Design review of the part built by this model. Coordinates are the model's own, in mm. Coordinates: 2 decimals unless noted, no trailing zeros. Order: outer loops, then holes, each group sorted by start corner. A loop starts at its lowest first (then second) coordinate and runs counter-clockwise, first axis right, second up. Notation, with made-up numbers: M -15.75,77 L 9.25,77 A20 ccw 9.25,99 Z; hole C 12.5,-29.75 d6. An arc over 180 degrees is marked long. Answer in a Markdown table with one row per item.
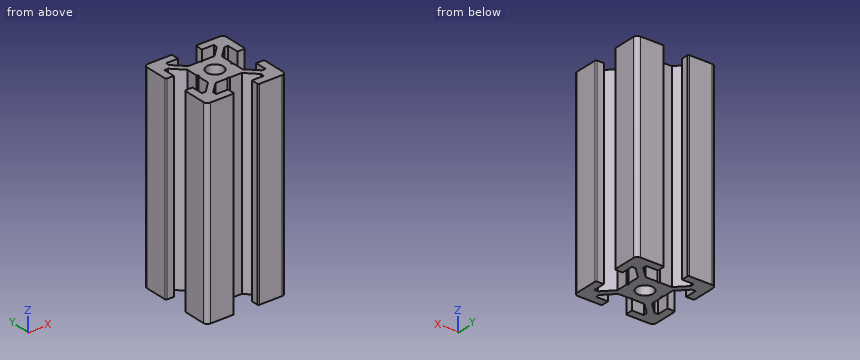
from build123d import *

# Parameters (mm, degrees)
SKETCH1_R           = 2.1
BOSS_EXTRUDE1_DEPTH = 50


with BuildPart() as part:
    # Sketch1 → Boss-Extrude1 (new body)
    with BuildSketch(Plane.XY):
        with BuildLine():
            Line((3.3, 4.360660172), (6.000039828, 7.0607))
            Line((6.000039828, 7.0607), (6.000039828, 8))
            Line((6.000039828, 8), (3.000039828, 8))
            Line((3.000039828, 8), (3.000039828, 9.7))
            ThreePointArc((3.000039828, 9.7), (3.087907794, 9.912132034), (3.300039828, 10))
            Line((3.300039828, 10), (9, 10))
            ThreePointArc((9, 10), (9.707106781, 9.707106781), (10, 9))
            Line((10, 9), (10, 3.300039828))
            ThreePointArc((10, 3.300039828), (9.912132034, 3.087907794), (9.7, 3.000039828))
            Line((9.7, 3.000039828), (8, 3.000039828))
            Line((8, 3.000039828), (8, 6.000039828))
            Line((8, 6.000039828), (7.0607, 6.000039828))
            Line((7.0607, 6.000039828), (4.360660172, 3.3))
            Line((4.360660172, 3.3), (4.360660172, 0.3))
            Line((4.360660172, 0.3), (4.060660172, 0))
            Line((4.060660172, 0), (4.360660172, -0.3))
            Line((4.360660172, -0.3), (4.360660172, -3.3))
            Line((4.360660172, -3.3), (7.0607, -6.000039828))
            Line((7.0607, -6.000039828), (8, -6.000039828))
            Line((8, -6.000039828), (8, -3.000039828))
            Line((8, -3.000039828), (9.7, -3.000039828))
            ThreePointArc((9.7, -3.000039828), (9.912132034, -3.087907794), (10, -3.300039828))
            Line((10, -3.300039828), (10, -9))
            ThreePointArc((10, -9), (9.707106781, -9.707106781), (9, -10))
            Line((9, -10), (3.300039828, -10))
            ThreePointArc((3.300039828, -10), (3.087907794, -9.912132034), (3.000039828, -9.7))
            Line((3.000039828, -9.7), (3.000039828, -8))
            Line((3.000039828, -8), (6.000039828, -8))
            Line((6.000039828, -8), (6.000039828, -7.0607))
            Line((6.000039828, -7.0607), (3.3, -4.360660172))
            Line((3.3, -4.360660172), (0.3, -4.360660172))
            Line((0.3, -4.360660172), (0, -4.060660172))
            Line((0, -4.060660172), (-0.3, -4.360660172))
            Line((-0.3, -4.360660172), (-3.3, -4.360660172))
            Line((-3.3, -4.360660172), (-6.000039828, -7.0607))
            Line((-6.000039828, -7.0607), (-6.000039828, -8))
            Line((-6.000039828, -8), (-3.000039828, -8))
            Line((-3.000039828, -8), (-3.000039828, -9.7))
            ThreePointArc((-3.000039828, -9.7), (-3.087907794, -9.912132034), (-3.300039828, -10))
            Line((-3.300039828, -10), (-9, -10))
            ThreePointArc((-9, -10), (-9.707106781, -9.707106781), (-10, -9))
            Line((-10, -9), (-10, -3.300039828))
            ThreePointArc((-10, -3.300039828), (-9.912132034, -3.087907794), (-9.7, -3.000039828))
            Line((-9.7, -3.000039828), (-8, -3.000039828))
            Line((-8, -3.000039828), (-8, -6.000039828))
            Line((-8, -6.000039828), (-7.0607, -6.000039828))
            Line((-7.0607, -6.000039828), (-4.360660172, -3.3))
            Line((-4.360660172, -3.3), (-4.360660172, -0.3))
            Line((-4.360660172, -0.3), (-4.060660172, 0))
            Line((-4.060660172, 0), (-4.360660172, 0.3))
            Line((-4.360660172, 0.3), (-4.360660172, 3.3))
            Line((-4.360660172, 3.3), (-7.0607, 6.000039828))
            Line((-7.0607, 6.000039828), (-8, 6.000039828))
            Line((-8, 6.000039828), (-8, 3.000039828))
            Line((-8, 3.000039828), (-9.7, 3.000039828))
            ThreePointArc((-9.7, 3.000039828), (-9.912132034, 3.087907794), (-10, 3.300039828))
            Line((-10, 3.300039828), (-10, 9))
            ThreePointArc((-10, 9), (-9.707106781, 9.707106781), (-9, 10))
            Line((-9, 10), (-3.300039828, 10))
            ThreePointArc((-3.300039828, 10), (-3.087907794, 9.912132034), (-3.000039828, 9.7))
            Line((-3.000039828, 9.7), (-3.000039828, 8))
            Line((-3.000039828, 8), (-6.000039828, 8))
            Line((-6.000039828, 8), (-6.000039828, 7.0607))
            Line((-6.000039828, 7.0607), (-3.3, 4.360660172))
            Line((-3.3, 4.360660172), (-0.3, 4.360660172))
            Line((-0.3, 4.360660172), (0, 4.060660172))
            Line((0, 4.060660172), (0.3, 4.360660172))
            Line((0.3, 4.360660172), (3.3, 4.360660172))
        make_face()
        Circle(SKETCH1_R, mode=Mode.SUBTRACT)
    extrude(amount=BOSS_EXTRUDE1_DEPTH)


solid = part.part
(1) Add section A-A, the plane y = -1. Give the boundary of the cut face in (x, z).
Return value:
| item | result |
|---|---|
| outline | M -4.36,0 L -1.85,0 L -1.85,50 L -4.36,50 Z; M 1.85,0 L 4.36,0 L 4.36,50 L 1.85,50 Z |
(2) Insertion check: pin 1 Ø0.9 at (y, z) = (-2.5, 34) entering from -X; pin 2 Ø0.9 at (x, z) = (-2, 29.5) entering from +Y; pin 3 Ø0.9 at (x, z) = (2, 37) entering from -Y. Each pin has a flat end and moves straight along its axis. Give the tip position at first contact, or say it passes through.
Return value:
| item | result |
|---|---|
| pin 1 | stops at x = -4.36 |
| pin 2 | stops at y = 4.36 |
| pin 3 | stops at y = -4.36 |
(3) For line 1 along X through (y, z) = (-9, 45.5); line 2 along X through (y, z) = (-7.5, 41); line 3 along Y through (x, z) = (-5, 29), list the stretches that pass through material, from the lowest coordinate up. Write a range as from..to.
Return value:
| item | result |
|---|---|
| line 1 | x = -10..-3, 3..10 |
| line 2 | x = -10..-6, 6..10 |
| line 3 | y = -10..-8, -6.06..-3.94, 3.94..6.06, 8..10 |
